Autodesk Inventor part; units mm, degrees
ref_plane "YZ Plane" through (0, 0, 0) normal (1, 0, 0) x (0, 1, 0)
ref_plane "XZ Plane" through (0, 0, 0) normal (0, 1, 0) x (-1, 0, 0)
ref_plane "XY Plane" through (0, 0, 0) normal (0, 0, 1) x (1, 0, 0)
sketch "Sketch1" plane through (0, 0, 0) normal (0, 0, 1) x (1, 0, 0)
  circle A0 centre (0, 0) radius 7.75
  circle A1 centre (0, 0) radius 9.75
  circle A2 centre (0, 0) radius 6.75
  circle A3 centre (0, 0) radius 14.75
  dimension "d0" = 15.5
  dimension "d1" = 2
  dimension "d2" = 1
  dimension "d5" = 5
extrude "Extrusion1" add sketch "Sketch1" against normal blind 5 contours A0
extrude "Extrusion2" add sketch "Sketch1" along normal blind 2 contours A0 | A1 | A3
fillet "Fillet1" radius 2 1 edges at (-14.75, 0, 0)
sketch "Sketch2" plane through (0, 0, 2) normal (0, 0, 1) x (1, 0, 0)
  circle A0 centre (0, 0) radius 12.75
  circle A1 centre (0, 0) radius 6.75
  dimension "d9" = 25.5
  dimension "d10" = 13.5
extrude "Extrusion3" add sketch "Sketch2" along normal blind 2
sketch "Sketch3" plane through (0, 0, 4) normal (0, 0, 1) x (1, 0, 0)
  circle A0 centre (0, 0) radius 6.75
  circle A1 centre (0, 0) radius 9.75
  dimension "d13" = 3
extrude "Extrusion4" add sketch "Sketch3" along normal blind 5
sketch "Sketch4" plane through (0, 0, 4) normal (0, 0, 1) x (1, 0, 0)
  circle A0 centre (0, 0) radius 9.75
  circle A1 centre (0, 0) radius 12.75
  line L0 (0, 20.65) -> (0, -20.65) construction
  circle A2 centre (0, 0) radius 9.75 construction
  line L1 (0, 9.75) -> (0, 12.75) construction
  line L2 (0, 11.25) -> (0.6069, 11.25) construction
  dimension "d27" = 25.5
hole "Hole1" at (0, 11.25, 4) direction (0, 0, -1) diameter 2 depth 3 tip angle 118
pattern_circular "Circular Pattern1" count 8 over 360 about axis through (0, 0, 0) along (0, 0, -1) of "Hole1"
properties part number "X-Ray Tube Output" material "Aluminum 6061"
Work out the finished part from the listing and answer in its coordinate system (mm). A direction names the side the tool comes from. Give positions to 0.01 mm unless a question says otherwise; leave off trailing zeros. Loops run counter-clockwise (first coordinate to the right, second up) from the corner with the lowest first, then second, coordinate; pieces in that order, holes last. Notation, with made-up numbers: (57, 74.25) -> (63, 74.25) arc R35 cw to (63, 111.25) -> close; hole circle Ø8 at (19, 88.25). An arc over 180 degrees is marked (long way). Use a Markdown table: item, result. Add a question column.
1) The part is cut by section A-A, the plane z = 8.25. Determine the outline of the cut face in (x, y), plus the area to 3 significant figures.
2) Which of the six approach directions +Z, -Z, +X, -X, +Y, -Y give full straight-line access (tool end or side, diameter ignored) to faces 1 (the flat face through (2, 7, 9)), 2 (the cylindrical face through (0.61, 12.04, 2.48))?
3) The part is cut by section C-C, the plane z = -3.5. Determine the outline of the cut face in (x, y).
4) The part is cut by section B-B, the plane z = 1.5. Count the separate pieces of the cut face and the enclosed holes in it, plus the area to 3 significant figures.
5) Each of these flat-tipped pins is pushed along its axis until it touches: P1, Ø1.2, axis at x = 0, y = 11.25, coming from the -Z side; P2, Ø1.8, axis at x = -7.95, y = -7.95, coming from the +Z side; P3, Ø1.2, axis at x = -7.95, y = 7.95, coming from the +Z side. Where does it stop, or does it pass through?
6) For a pull along Y with two mould halves and no side action, classify faces 3 (the cylindrical face through (-8.256, -7.001, 2.479)), 4 (the cylindrical face through (-1.269, -9.667, 6.465)), 5 (the flat face through (-5, 9, 4)) as +Y half, -Y half, draft (parallel to the pull), parting line (faces both ways), or undercut.
7) Consider line 1 along Y through (x, z) = (7.25, 3.75); line 2 along Z through (x, y) = (-10, -5.5); line 3 along Y through (x, z) = (-11.25, 1.6). Determine where each line is inside the solid, lowest interval first.
Reported:
| question | item | result |
|---|---|---|
| 1 | outline | circle Ø19.5 at (0, 0); hole circle Ø13.5 at (0, 0) |
| 1 | area | 156 mm^2 |
| 2 | face 1 | +Z, +X, -X, +Y, -Y |
| 2 | face 2 | +Z |
| 3 | outline | circle Ø15.5 at (0, 0); hole circle Ø13.5 at (0, 0) |
| 4 | separate pieces | 1 |
| 4 | enclosed holes | 9 |
| 4 | area | 509 mm^2 |
| 5 | P1 | stops at z = 0 |
| 5 | P2 | stops at z = 0.94 |
| 5 | P3 | stops at z = 0.76 |
| 6 | face 3 | undercut |
| 6 | face 4 | parting line |
| 6 | face 5 | draft |
| 7 | line 1 | y = -10.49 to -8.66, -7.25 to 7.25, 8.66 to 10.49 |
| 7 | line 2 | z = 0 to 4 |
| 7 | line 3 | y = -9.48 to -1, 1 to 9.48 |
